Job drawing, mm, ordinate dimensions from the low corner. One solid piece. A direction names the side the tool comes from. Round coordinates to 2 decimals unless told otherwise and drop trailing zeros. Loops run counter-clockwise (first coordinate to the right, second up) from the corner with the lowest first, then second, coordinate; pieces in that order, holes last. Notation, with made-up numbers: M -14.75,87.5 L 0.25,87.5 A20 ccw 0.25,107.5 Z; hole C -15,43.25 d2. An arc over 180 degrees is marked long. Use a Markdown table: item, result. Add a question column.
(1) Which spindle directions (+Z, -Z, +X, -X, +Y, -Y) get a long thin tool onto all of the face, cutting with end or side? Do the marked faces 1 and 2. Say none if no direction does.
(2) Flat gauge pins, fed straight in: P1, Ø4, axis at x = 39, y = 39, coming from the -Z side; P2, Ø3, axis at x = 7, y = 7, coming from the -Z side. Where does each tip first touch, or does it go through?
(3) Wall check: L1, parallel to X at y = 12.5, z = 2.5; L2, parallel to Y at x = 39, z = 5.85. Give the ranges that are in metal, low to high.
(4) Band-saw the part on A-A, the plane z = 6.25. Write the cut outline in (x, y), and give its area (3 significant figures).
(5) Band-saw the part on C-C, the plane y = 17. Write the cut outline in (x, z).
(6) Two-plate mould, pull along X, no slides. Class the marked faces 3, 4 and 5: released by +X, released by -X, zero draft, split by the parting line, or undercut.
(7) Band-saw the part on D-D, the plane y = 25. Write the cut outline in (x, z), and give its area (3 significant figures).
(8) Band-saw the part on B-B, the plane z = 1.75. Write the cut outline in (x, y).
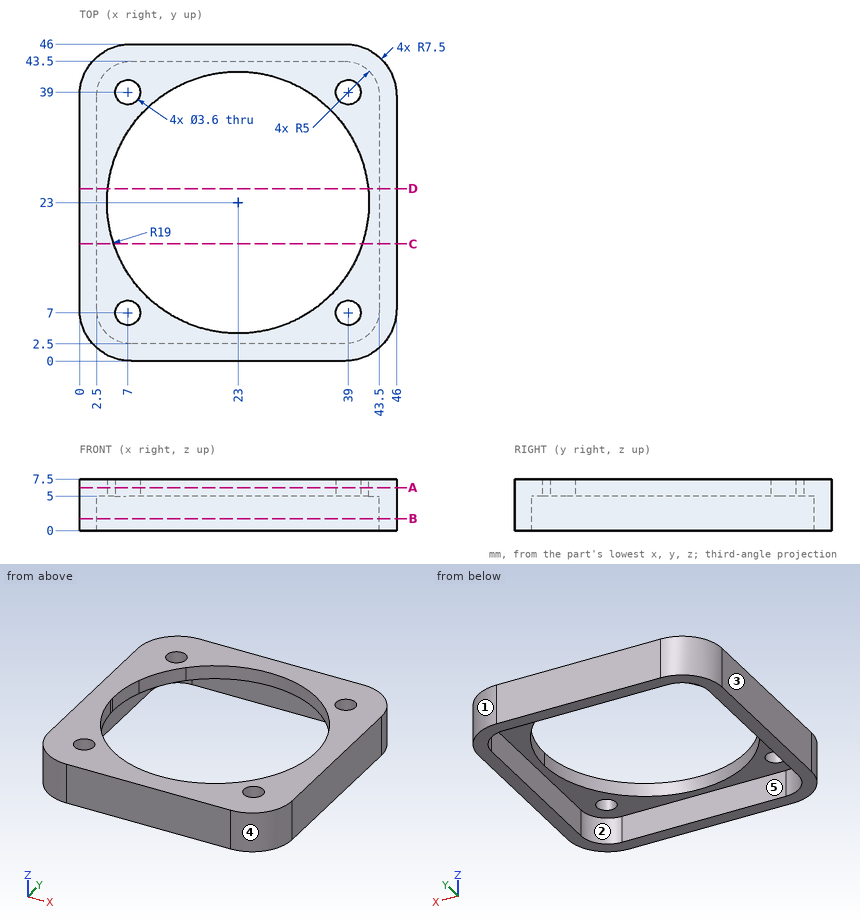
Return value:
| question | item | result |
|---|---|---|
| 1 | face 1 | +Z, -Z, +X, +Y |
| 1 | face 2 | -Z |
| 2 | P1 | z = 5 |
| 2 | P2 | through |
| 3 | L1 | 0 to 2.5, 43.5 to 46 |
| 3 | L2 | 0.02 to 5.2, 8.8 to 12.75, 33.25 to 37.2, 40.8 to 45.98 |
| 4 | outline | M 0,7.5 A7.5 ccw 7.5,0 L 38.5,0 A7.5 ccw 46,7.5 L 46,38.5 A7.5 ccw 38.5,46 L 7.5,46 A7.5 ccw 0,38.5 Z; hole C 23,23 d38; hole C 7,7 d3.6; hole C 7,39 d3.6; hole C 39,7 d3.6; hole C 39,39 d3.6 |
| 4 | area | 893 mm^2 |
| 5 | outline | M 0,0 L 2.5,0 L 2.5,5 L 4.97,5 L 4.97,7.5 L 0,7.5 Z; M 41.03,5 L 43.5,5 L 43.5,0 L 46,0 L 46,7.5 L 41.03,7.5 Z |
| 6 | face 3 | released by -X |
| 6 | face 4 | released by +X |
| 6 | face 5 | undercut |
| 7 | outline | M 0,0 L 2.5,0 L 2.5,5 L 4.11,5 L 4.11,7.5 L 0,7.5 Z; M 41.89,5 L 43.5,5 L 43.5,0 L 46,0 L 46,7.5 L 41.89,7.5 Z |
| 7 | area | 45.5 mm^2 |
| 8 | outline | M 0,7.5 A7.5 ccw 7.5,0 L 38.5,0 A7.5 ccw 46,7.5 L 46,38.5 A7.5 ccw 38.5,46 L 7.5,46 A7.5 ccw 0,38.5 Z; hole M 2.5,7.5 A5 ccw 7.5,2.5 L 38.5,2.5 A5 ccw 43.5,7.5 L 43.5,38.5 A5 ccw 38.5,43.5 L 7.5,43.5 A5 ccw 2.5,38.5 Z |
